Check sheet for the modelled part. Datum: model origin and axes. Units: mm. Face numbers are marked on the shaded views. Coordinates: 2 decimals unless noted, no trailing zeros. Write each loop counter-clockwise with the first axis right and the second up, starting at its lowest first coordinate (ties: lowest second). Pieces come first, ordered by that corner, then holes. Notation, with made-up numbers: (86, 87.5) - (138, 87.5) arc R15 cw to (138, 115.5) - close; hole circle Ø9 at (62, -24.5). An arc over 180 degrees is marked (long way). Answer as CSV lines item,"result". Start each with the question number.
from build123d import *

# Parameters (mm, degrees)
SKETCH1_W           = 37.846
SKETCH1_H           = 31.75
BOSS_EXTRUDE1_DEPTH = 7.874
SKETCH2_R           = 1.8415
CUT_EXTRUDE1_DEPTH  = 16.748


with BuildPart() as part:
    # Sketch1 → Boss-Extrude1 (new body, symmetric)
    with BuildSketch(Plane(origin=(0, 0, 0), x_dir=(1, 0, 0), z_dir=(0, 1, 0))):
        Rectangle(SKETCH1_W, SKETCH1_H)
    extrude(amount=BOSS_EXTRUDE1_DEPTH, both=True)

    # Sketch2 → Cut-Extrude1 (cut, through all)
    with BuildSketch(Plane.XZ.offset(7.874)):
        with Locations((-16.383, 13.335)):
            Circle(SKETCH2_R)
        with Locations((16.383, 13.335)):
            Circle(SKETCH2_R)
        with Locations((16.383, -13.335)):
            Circle(SKETCH2_R)
        with Locations((-16.383, -13.335)):
            Circle(SKETCH2_R)
    extrude(amount=-CUT_EXTRUDE1_DEPTH, mode=Mode.SUBTRACT)


solid = part.part
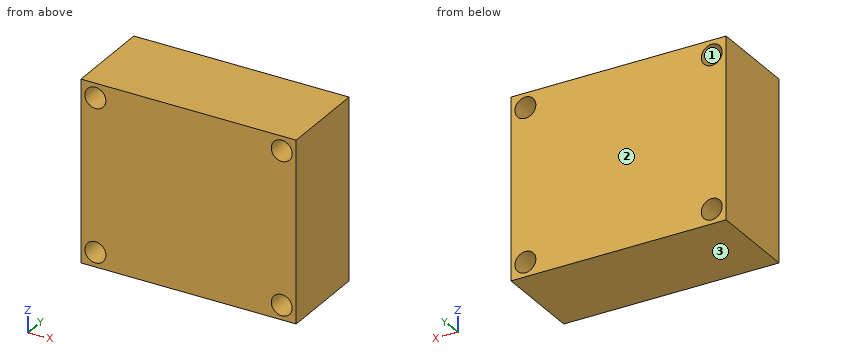
(1) Cross-section at A-A on x = 15. Record the boundary of the cut face in (y, z) (3 decimals), plus the area to 3 significant figures.
(2) Material ranges on probe 1 along X at (y, z) = (-2.5, 13.5); probe 2 along X at (y, z) = (3, 13); probe 3 along Z at (x, y) = (16, -4.25) (3 decimals), recorded low to high. Write a range as from..to.
(3) Release check for a two-part mould opening along Z. For the marked faces 1, 2 and 3 record: pulls with the +Z half, pulls with the -Z half, needs draft (parallel to the pull), parting line crosses it, or undercut.
(4) Cross-section at B-B on y = 1.75. Record the boundary of the cut face in (x, z) (1 decimal), plus the area to 3 significant figures.
Checked values:
1,outline,"(-7.874, -15.875) - (7.874, -15.875) - (7.874, -14.551) - (-7.874, -14.551) - close; (-7.874, -12.119) - (7.874, -12.119) - (7.874, 12.119) - (-7.874, 12.119) - close; (-7.874, 14.551) - (7.874, 14.551) - (7.874, 15.875) - (-7.874, 15.875) - close"
1,area,"423 mm^2"
2,probe 1,"-18.92..-18.22, -14.55..14.55, 18.22..18.92"
2,probe 2,"-18.92..-18.19, -14.57..14.57, 18.19..18.92"
2,probe 3,"-15.875..-15.136, -11.534..11.534, 15.136..15.875"
3,face 1,"undercut"
3,face 2,"needs draft"
3,face 3,"pulls with the -Z half"
4,outline,"(-18.9, -15.9) - (18.9, -15.9) - (18.9, 15.9) - (-18.9, 15.9) - close; hole circle Ø3.7 at (-16.4, -13.3); hole circle Ø3.7 at (-16.4, 13.3); hole circle Ø3.7 at (16.4, -13.3); hole circle Ø3.7 at (16.4, 13.3)"
4,area,"1,160 mm^2"
